```python
from build123d import *

# Parameters (mm, degrees)
F0_W      = 76.2
F0_H      = 50.8
F1_DEPTH  = 30.1625
F3_DEPTH  = 30.1625
F4_R      = 11.1125
F5_DEPTH  = 30.1625
F7_DEPTH  = 20.6375
F8_DEPTH  = 30.1625
F9_R      = 15.875
F10_DEPTH = 50.8
F12_DEPTH = 50.8


with BuildPart() as f1:
    # F0 (on Front) → F1 (new body)
    with BuildSketch(Plane.XZ):
        with Locations((6.8375896662, 9.2583434884)):
            Rectangle(F0_W, F0_H)
    extrude(amount=F1_DEPTH)

    # F2 (on face) → F3 (join)
    with BuildSketch(Plane(origin=(0, 0, 0), x_dir=(-1, 0, 0), z_dir=(0, 1, 0))):
        with BuildLine():
            Line((-44.9375896662, -16.1416565116), (-44.9375896662, 34.6583434884))
            ThreePointArc((-44.9375896662, 34.6583434884), (-70.3375896662, 9.2583434884), (-44.9375896662, -16.1416565116))
        make_face()
    extrude(amount=-F3_DEPTH)

    # F4 (on face) → F5 (cut)
    with BuildSketch(Plane.XZ.offset(30.1625)):
        with Locations((44.9375896662, 9.2583434884)):
            Circle(F4_R)
    extrude(amount=-F5_DEPTH, mode=Mode.SUBTRACT)

    # F6 (on face) → F7 (join)
    with BuildSketch(Plane.XZ.offset(30.1625)):
        with BuildLine():
            Line((-31.2624103338, 34.6583434884), (-12.2124103338, 34.6583434884))
            ThreePointArc((-12.2124103338, 34.6583434884), (-63.0124103338, 9.2583434884), (-12.2124103338, -16.1416565116))
            Line((-12.2124103338, -16.1416565116), (-31.2624103338, -16.1416565116))
            Line((-31.2624103338, -16.1416565116), (-31.2624103338, 34.6583434884))
        make_face()
        with BuildLine():
            ThreePointArc((-12.2124103338, -16.1416565116), (-2.8643470195, -4.9406881687), (0.4875896662, 9.2583434884))
            ThreePointArc((0.4875896662, 9.2583434884), (-2.8643470195, 23.4573751456), (-12.2124103338, 34.6583434884))
            Line((-12.2124103338, 34.6583434884), (-31.2624103338, 34.6583434884))
            Line((-31.2624103338, 34.6583434884), (-31.2624103338, -16.1416565116))
            Line((-31.2624103338, -16.1416565116), (-12.2124103338, -16.1416565116))
        make_face()
    extrude(amount=F7_DEPTH)

    # F8 (add): a face of the model
    f8_faces = [f1.faces().sort_by_distance(p)[0] for p in [
        (-42.7836943553, -30.1625, 9.2583434884),
    ]]
    extrude(f8_faces, amount=F8_DEPTH)

    # F9 (on face) → F10 (cut)
    with BuildSketch(Plane.XZ.offset(50.8)):
        with Locations((-31.2624103338, 9.2583434884)):
            Circle(F9_R)
    extrude(amount=-F10_DEPTH, mode=Mode.SUBTRACT)

    # F11 (on face) → F12 (cut)
    with BuildSketch(Plane.XZ.offset(50.8)):
        with BuildLine():
            Line((-11.3561255113, 14.0208434884), (-16.1186255113, 14.0208434884))
            ThreePointArc((-16.1186255113, 14.0208434884), (-15.5712789364, 11.6674969645), (-15.3874103338, 9.2583434884))
            ThreePointArc((-15.3874103338, 9.2583434884), (-15.5712789364, 6.8491900123), (-16.1186255113, 4.4958434884))
            Line((-16.1186255113, 4.4958434884), (-11.3561255113, 4.4958434884))
            Line((-11.3561255113, 4.4958434884), (-11.3561255113, 14.0208434884))
        make_face()
    extrude(amount=-F12_DEPTH, mode=Mode.SUBTRACT)


solid = f1.part
```
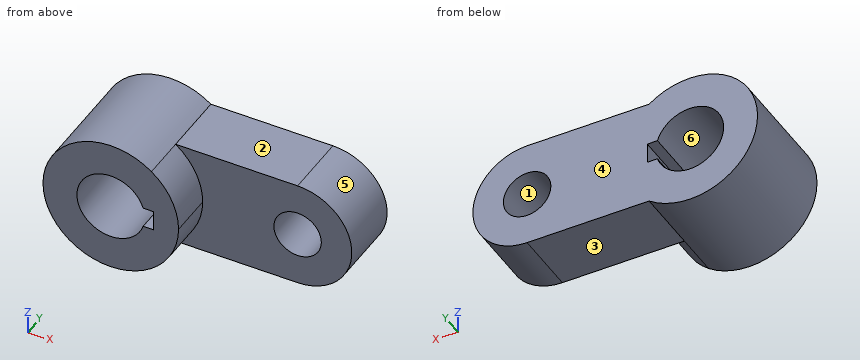
Source: CAD feature listing. Evaluate the final solid. Frame: model axes, mm. Face numbers are marked on the shaded views. A direction names the side the tool comes from. Coordinates: 2 decimals unless noted, no trailing zeros. Loops run counter-clockwise (first coordinate to the right, second up) from the corner with the lowest first, then second, coordinate; pieces in that order, holes last. Notation, with made-up numbers: (23, 61) -> (62, 61) arc R34 ccw to (62, 94) -> close; hole circle Ø2 at (65, 34.25). An arc over 180 degrees is marked (long way). One line per item, written item: value. Start each with the question number.
Q1. Set-up query: the marked faces 1, 2 and 3. Return all of +Z, -Z, +X, -X, +Y, -Y with unobstructed straight access to the full face (end or side cutting, diameter ignored); none if empty.
Q2. Section query B-B, the plane y = -26. Give the number of separate pieces and of enclosed holes in the cut face, and give its area (3 significant figures).
Q3. Section query D-D, the plane x = -34. Return the cut outline in (y, z).
Q4. Mould query, pull axis X, two halves, no side actions, for the marked faces 4, 5 and 6. Classes: pulls with the +X half, pulls with the -X half, needs draft (parallel to the pull), parting line crosses it, or undercut.
Q5. Section query C-C, the plane z = 0. Return the cut outline in (x, y), and give its area (3 significant figures).
Q6. Contact query for flat-ended pins moving along their axis: P1, Ø5, axis at x = -14, y = -29.5, coming from the -Z side; P2, Ø3, axis at x = 38.5, z = 29.5, coming from the -Y side; P3, Ø24, axis at x = 13, y = -20.5, coming from the +Z side; P4, Ø12, axis at x = -39, z = 17.5, coming from the +Y side. Output: stop coordinate, or through.
Q7. Line query: line 1 along X through (y, z) = (-17, 7); line 2 along X through (y, z) = (-38, 8.5); line 3 along Z through (x, y) = (-11.5, -16). Output: solid intervals per line, ascending.
Q8. Section query A-A, the plane y = -46.5. Return the cut outline in (x, z) (3 decimals), and give its area (3 significant figures).
Results:
1. face 1: +Y, -Y
1. face 2: +Z, +X, +Y, -Y
1. face 3: -Z, +X, +Y, -Y
2. separate pieces: 1
2. enclosed holes: 2
2. area: 5,410 mm^2
3. outline: (-50.8, -22.37) -> (0, -22.37) -> (0, -6.38) -> (-50.8, -6.38) -> close; (-50.8, 24.9) -> (0, 24.9) -> (0, 40.89) -> (-50.8, 40.89) -> close
4. face 4: needs draft
4. face 5: pulls with the +X half
4. face 6: undercut
5. outline: (-61.63, -50.8) -> (-44.16, -50.8) -> (-44.16, 0) -> (-61.63, 0) -> close; (-18.37, -50.8) -> (-0.89, -50.8) -> (-0.89, -30.16) -> (38.79, -30.16) -> (38.79, 0) -> (-18.37, 0) -> close; (51.08, -30.16) -> (68.59, -30.16) -> (68.59, 0) -> (51.08, 0) -> close
5. area: 3,500 mm^2
6. P1: z = -18.85
6. P2: y = -30.16
6. P3: z = 34.66
6. P4: y = 0
7. line 1: -62.93 to -46.98, -11.36 to 34.06, 55.82 to 70.24
7. line 2: -63 to -47.12, -11.36 to 0.48
7. line 3: -16.14 to 4.5, 14.02 to 34.66
8. outline: circle Ø63.5 at (-31.262, 9.258); hole (-16.119, 4.496) -> (-11.356, 4.496) -> (-11.356, 14.021) -> (-16.119, 14.021) arc R15.875 ccw (long way) to start
8. area: 2,330 mm^2
